Job drawing, mm, ordinate dimensions from the low corner. One solid piece. Give positions to 0.01 mm unless a question says otherwise; leave off trailing zeros. Write each loop counter-clockwise with the first axis right and the second up, starting at its lowest first coordinate (ties: lowest second). Pieces come first, ordered by that corner, then holes. Notation, with made-up numbers: M 67.25,1.5 L 76.25,1.5 A13 ccw 76.25,21.5 Z; hole C 30.25,-20 d6. An arc over 180 degrees is marked long. Answer as CSV lines item,"result". Start each with the question number.
1) Slice it at D-D, the plane x = 22. Give the cut face in (y, z) (1 decimal), plus the area to 3 significant figures.
2) Slice it at B-B, the plane x = 33. Give the number of separate pieces and of enclosed holes in the cut face, plus the area to 3 significant figures.
3) Pin check, flat tips, straight feed: pin 1 Ø6.5 at (x, y) = (57, 32) entering from +Z; pin 2 Ø1.5 at (x, z) = (16.5, 5) entering from +Y; pin 3 Ø2.5 at (x, z) = (31, 8) entering from -Y; pin 4 Ø3 at (x, y) = (7, 32) entering from +Z. Stop position of each tip, or through.
4) Wall check: line 1 along Z through (x, y) = (9, 10); line 2 along X through (y, z) = (31.5, 0.75) (1 decimal); line 3 along Y through (x, z) = (19, 9.75) (1 decimal). Give the ranges that are in metal, low to high. Write a range as from..to.
5) Slice it at A-A, the plane y = 39. Give the cut face in (x, z) (1 decimal).
6) Mould opens along X. For the marked faces 1, 2 and 3 say: pulls with the +X half, pulls with the -X half, needs draft (parallel to the pull), parting line crosses it, or undercut.
7) Slice it at C-C, the plane z = 3. Give the cut face in (x, y) (1 decimal).
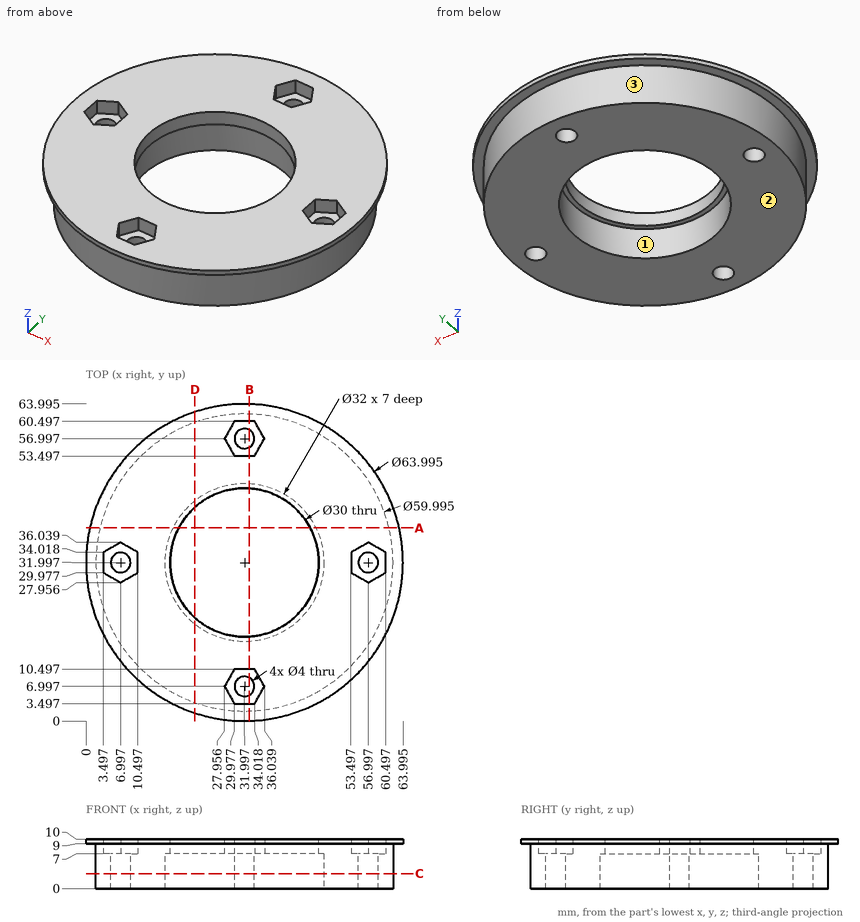
Found:
1,outline,"M 1.6,9 L 3.7,9 L 3.7,0 L 19.5,0 L 19.5,7 L 20.8,7 L 20.8,10 L 1.6,10 Z; M 43.2,7 L 44.5,7 L 44.5,0 L 60.3,0 L 60.3,9 L 62.4,9 L 62.4,10 L 43.2,10 Z"
1,area,"328 mm²"
2,separate pieces,"4"
2,enclosed holes,"0"
2,area,"200 mm²"
3,pin 1,"z = 7"
3,pin 2,"y = 58.12"
3,pin 3,"y = 0"
3,pin 4,"through"
4,line 1,"9..10"
4,line 2,"2..5.1, 8.9..16, 48..55.1, 58.9..62"
4,line 3,"2.8..24.5, 39.5..61.2"
5,outline,"M 0.8,9 L 2.8,9 L 2.8,0 L 17.6,0 L 17.6,7 L 18.7,7 L 18.7,10 L 0.8,10 Z; M 45.3,7 L 46.4,7 L 46.4,0 L 61.2,0 L 61.2,9 L 63.2,9 L 63.2,10 L 45.3,10 Z"
6,face 1,"undercut"
6,face 2,"needs draft"
6,face 3,"parting line crosses it"
7,outline,"C 32,32 d60; hole C 7,32 d4; hole C 32,32 d32; hole C 32,7 d4; hole C 32,57 d4; hole C 57,32 d4"
